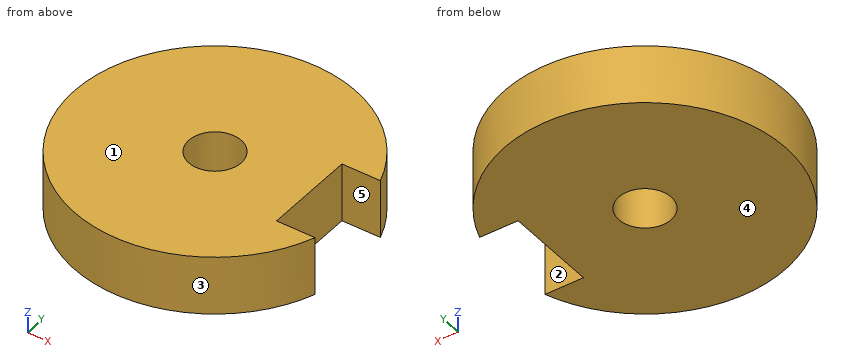
from build123d import *

# Parameters (mm, degrees)
SKETCH1_R           = 7.585
SKETCH1_R_2         = 1.415
BOSS_EXTRUDE1_DEPTH = 3.175
SKETCH2_W           = 2.5
SKETCH2_H           = 5
CUT_EXTRUDE1_DEPTH  = 3.175


with BuildPart() as part:
    # Sketch1 → Boss-Extrude1 (new body)
    with BuildSketch(Plane.XY):
        Circle(SKETCH1_R)
        Circle(SKETCH1_R_2, mode=Mode.SUBTRACT)
    extrude(amount=BOSS_EXTRUDE1_DEPTH)

    # Sketch2 → Cut-Extrude1 (cut)
    with BuildSketch(Plane.XY.offset(3.175)):
        with Locations((6.335, 0)):
            Rectangle(SKETCH2_W, SKETCH2_H)
    extrude(amount=-CUT_EXTRUDE1_DEPTH, mode=Mode.SUBTRACT)


solid = part.part
Check sheet for the modelled part. Datum: model origin and axes. Units: mm. Face numbers are marked on the shaded views. A direction names the side the tool comes from. Coordinates: 2 decimals unless noted, no trailing zeros. Loops run counter-clockwise (first coordinate to the right, second up) from the corner with the lowest first, then second, coordinate; pieces in that order, holes last. Notation, with made-up numbers: (-0.5, 14) -> (47.5, 14) arc R22 ccw to (47.5, 28) -> close; hole circle Ø11 at (-36, 80). An arc over 180 degrees is marked (long way). Write item = value, one per line. Start each with the question number.
1. Draft check along Y on the marked faces 3, 4 and 5. Enter one of: released by +Y, released by -Y, zero draft, split by the parting line, or undercut.
2. Section check B-B on y = 0. Record the cut outline in (x, z) (3 decimals), then the cut area to 3 significant figures.
3. Section check C-C on z = 2.3. Record the cut outline in (x, y) (3 decimals).
4. Section check D-D on y = 4. Record the cut outline in (x, z) (3 decimals).
5. Tool access check on the marked faces 1 and 2. Record the directions out of +Z, -Z, +X, -X, +Y, -Y that give a thin tool (end or side, any length) a straight path to the whole face; none if there is none.
6. Depth check by flat-ended pin: P1, Ø1, axis at x = -5.5, z = 2.5, coming from the +Y side; P2, Ø1, axis at y = 0.5, z = 1, coming from the +X side (3 decimals); P3, Ø1, axis at x = 6.5, z = 1, coming from the +Y side; P4, Ø3.5, axis at x = 0, y = 0, coming from the -Z side. Enter the tip coordinate at first touch or a pass-through.
7. Material ranges on line 1 (Y direction, x = 0, z = 2.4) (3 decimals); line 2 (Y direction, x = 1, z = 2.8); line 3 (X direction, y = 0.25, z = 0.7) (3 decimals), recorded low to high.
8. Section check A-A on x = 0. Record the cut outline in (y, z) (3 decimals), then the cut area to 3 significant figures.
Responses:
q1.face_3 = split by the parting line
q1.face_4 = zero draft
q1.face_5 = undercut
q2.outline = (-7.585, 0) -> (-1.415, 0) -> (-1.415, 3.175) -> (-7.585, 3.175) -> close; (1.415, 0) -> (5.085, 0) -> (5.085, 3.175) -> (1.415, 3.175) -> close
q2.area = 31.2 mm2
q3.outline = (5.085, -2.5) -> (5.085, 2.5) -> (7.161, 2.5) arc R7.585 ccw (long way) to (7.161, -2.5) -> close; hole circle Ø2.83 at (0, 0)
q4.outline = (-6.445, 0) -> (6.445, 0) -> (6.445, 3.175) -> (-6.445, 3.175) -> close
q5.face_1 = +Z, +X, -X, +Y, -Y
q5.face_2 = +Z, -Z, +X
q6.P1 = 5.7
q6.P2 = 5.085
q6.P3 = 4.64
q6.P4 = 0
q7.line_1 = -7.585 to -1.415, 1.415 to 7.585
q7.line_2 = -7.52 to -1, 1 to 7.52
q7.line_3 = -7.581 to -1.393, 1.393 to 5.085
q8.outline = (-7.585, 0) -> (-1.415, 0) -> (-1.415, 3.175) -> (-7.585, 3.175) -> close; (1.415, 0) -> (7.585, 0) -> (7.585, 3.175) -> (1.415, 3.175) -> close
q8.area = 39.2 mm2
